from build123d import *

# Parameters (mm, degrees)
SKETCH1_W               = 106
SKETCH1_H               = 57
BOSS_EXTRUDE1_DEPTH     = 1.5
SKETCH2_W               = 3
SKETCH2_H               = 22.5
SKETCH2_W_2             = 40
SKETCH2_H_2             = 3
CUT_EXTRUDE1_DEPTH      = 2.5
CUT_EXTRUDE1_DEPTH_BACK = 2.5
SKETCH4_W               = 15
SKETCH4_H               = 9
BOSS_EXTRUDE2_DEPTH     = 1.5
FILLET1_R               = 2
CUT_EXTRUDE2_DEPTH      = 2.5
CUT_EXTRUDE2_DEPTH_BACK = 2.5
SKETCH5_R               = 1.5
CUT_EXTRUDE3_DEPTH      = 2.5
CUT_EXTRUDE3_DEPTH_BACK = 2.5
FILLET2_R               = 5
SKETCH6_R               = 1.5
CUT_EXTRUDE4_DEPTH      = 2.5
CUT_EXTRUDE4_DEPTH_BACK = 2.5


with BuildPart() as part:
    # Sketch1 → Boss-Extrude1 (new body, symmetric)
    with BuildSketch(Plane(origin=(0, 0, 0), x_dir=(1, 0, 0), z_dir=(0, 1, 0))):
        Rectangle(SKETCH1_W, SKETCH1_H)
    extrude(amount=BOSS_EXTRUDE1_DEPTH, both=True)

    # Sketch2 → Cut-Extrude1 (cut, two sides)
    with BuildSketch(Plane(origin=(0, 0, 0), x_dir=(1, 0, 0), z_dir=(0, 1, 0))) as cut_extrude1_sk:
        with Locations((-51.5, 17.25)):
            Rectangle(SKETCH2_W, SKETCH2_H)
        with Locations((51.5, 17.25)):
            Rectangle(SKETCH2_W, SKETCH2_H)
        with Locations((0, -27)):
            Rectangle(SKETCH2_W_2, SKETCH2_H_2)
    extrude(amount=CUT_EXTRUDE1_DEPTH, mode=Mode.SUBTRACT)
    extrude(cut_extrude1_sk.sketch, amount=-CUT_EXTRUDE1_DEPTH_BACK, mode=Mode.SUBTRACT)

    # Sketch4 → Boss-Extrude2 (add, symmetric)
    with BuildSketch(Plane(origin=(0, 0, 0), x_dir=(1, 0, 0), z_dir=(0, 1, 0))):
        with Locations((0, 33)):
            Rectangle(SKETCH4_W, SKETCH4_H)
    extrude(amount=BOSS_EXTRUDE2_DEPTH, both=True)

    # Fillet1
    fillet1_edges = [part.edges().sort_by_distance(p)[0] for p in [
        (-7.5, 0, -37.5),
        (-7.5, 0, -28.5),
        (7.5, 0, -28.5),
        (7.5, 0, -37.5),
    ]]
    fillet(fillet1_edges, radius=FILLET1_R)

    # Sketch3 → Cut-Extrude2 (cut, two sides)
    with BuildSketch(Plane(origin=(0, 0, 0), x_dir=(1, 0, 0), z_dir=(0, 1, 0))) as cut_extrude2_sk:
        with BuildLine():
            Line((-1.5, -25.5), (1.5, -25.5))
            Line((1.5, -25.5), (1.5, -21.5))
            Line((1.5, -21.5), (2.8, -21.5))
            Line((2.8, -21.5), (2.8, -19.23))
            Line((2.8, -19.23), (1.5, -19.23))
            Line((1.5, -19.23), (1.5, -14.5))
            ThreePointArc((1.5, -14.5), (1.207106781, -13.792893219), (0.5, -13.5))
            Line((0.5, -13.5), (-0.5, -13.5))
            ThreePointArc((-0.5, -13.5), (-1.207106781, -13.792893219), (-1.5, -14.5))
            Line((-1.5, -14.5), (-1.5, -19.23))
            Line((-1.5, -19.23), (-2.8, -19.23))
            Line((-2.8, -19.23), (-2.8, -21.5))
            Line((-2.8, -21.5), (-1.5, -21.5))
            Line((-1.5, -21.5), (-1.5, -25.5))
        make_face()
    extrude(amount=CUT_EXTRUDE2_DEPTH, mode=Mode.SUBTRACT)
    extrude(cut_extrude2_sk.sketch, amount=-CUT_EXTRUDE2_DEPTH_BACK, mode=Mode.SUBTRACT)

    # Sketch5 → Cut-Extrude3 (cut, two sides)
    with BuildSketch(Plane(origin=(0, 0, 0), x_dir=(1, 0, 0), z_dir=(0, 1, 0))) as cut_extrude3_sk:
        with Locations((0, 33)):
            Circle(SKETCH5_R)
    extrude(amount=CUT_EXTRUDE3_DEPTH, mode=Mode.SUBTRACT)
    extrude(cut_extrude3_sk.sketch, amount=-CUT_EXTRUDE3_DEPTH_BACK, mode=Mode.SUBTRACT)

    # Fillet2
    fillet2_edges = [part.edges().sort_by_distance(p)[0] for p in [
        (53, 0, 28.5),
        (-53, 0, 28.5),
    ]]
    fillet(fillet2_edges, radius=FILLET2_R)

    # Sketch6 → Cut-Extrude4 (cut, two sides)
    with BuildSketch(Plane(origin=(0, 0, 0), x_dir=(1, 0, 0), z_dir=(0, 1, 0))) as cut_extrude4_sk:
        with Locations((-21, -15)):
            Circle(SKETCH6_R)
        with Locations((-12.4, -15)):
            Circle(SKETCH6_R)
        with Locations((12.4, -15)):
            Circle(SKETCH6_R)
        with Locations((21, -15)):
            Circle(SKETCH6_R)
    extrude(amount=CUT_EXTRUDE4_DEPTH, mode=Mode.SUBTRACT)
    extrude(cut_extrude4_sk.sketch, amount=-CUT_EXTRUDE4_DEPTH_BACK, mode=Mode.SUBTRACT)


solid = part.part
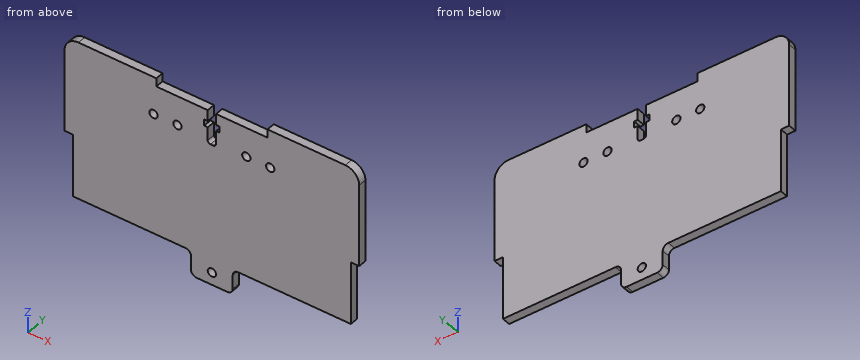
Input: part model. Units: mm. Frame: model coordinates. Coordinates: 2 decimals unless noted, no trailing zeros. Loops run counter-clockwise (first coordinate to the right, second up) from the corner with the lowest first, then second, coordinate; pieces in that order, holes last.
Q1. Contact query for flat-ended pins moving along their axis: pin 1 (1.5 mm diameter, centred on x = 10, y = -0.5, fed in from +Z); pin 2 (1.5 mm diameter, centred on y = -0.5, z = 27, fed in from -X); pin 3 (0.9 mm diameter, centred on y = -0.5, z = 24.5, fed in from +X). Output: stop coordinate, or through.
Q2. Cut plane C-C (y = 0.05). Give the number of separate pieces and of enclosed holes in the cut face, then the cut area to 3 significant figures.
Q3. Cut plane D-D (z = -19). Output: boundary loops of the cut face in (x, y), then the cut area to 3 significant figures.
Q4. Material intervals for line 1 (X direction, y = 0.15, z = 15); line 2 (Z direction, x = 21, y = 0.9); line 3 (Z direction, x = 12.4, y = 0.75), sorted ascending.
Q5. Cut plane B-B (x = -21). Output: boundary loops of the cut face in (y, z).
Q6. Cut plane A-A (z = -33). Output: boundary loops of the cut face in (x, y).
Working result:
1. pin 1: stops at z = 25.5
1. pin 2: stops at x = -52.18
1. pin 3: stops at x = 52.97
2. separate pieces: 1
2. enclosed holes: 5
2. area: 5,830 mm2
3. outline: (-50, -1.5) - (50, -1.5) - (50, 1.5) - (-50, 1.5) - close
3. area: 300 mm2
4. line 1: x = -53 to -22.5, -19.5 to -13.9, -10.9 to -1.5, 1.5 to 10.9, 13.9 to 19.5, 22.5 to 53
4. line 2: z = -28.5 to 13.5, 16.5 to 28.5
4. line 3: z = -28.5 to 13.5, 16.5 to 25.5
5. outline: (-1.5, -28.5) - (1.5, -28.5) - (1.5, 13.5) - (-1.5, 13.5) - close; (-1.5, 16.5) - (1.5, 16.5) - (1.5, 28.5) - (-1.5, 28.5) - close
6. outline: (-7.5, -1.5) - (-1.5, -1.5) - (-1.5, 1.5) - (-7.5, 1.5) - close; (1.5, -1.5) - (7.5, -1.5) - (7.5, 1.5) - (1.5, 1.5) - close
